from build123d import *

# Parameters (mm, degrees)
BOSS_EXTRUDE1_DEPTH = 20
SHELL1_T            = -5


with BuildPart() as part:
    # Sketch2 → Boss-Extrude1 (new body)
    with BuildSketch(Plane.XY):
        Polygon((-61.336329504, -46.981018343), (97.131391098, -46.981018343), (97.131391098, 27.778459258), (71.904316974, 27.778459258), (71.904316974, 47.185045125), (46.299911218, 47.185045125), (46.299911218, 27.739957348), (-61.336329504, 27.739957348), align=None)
    extrude(amount=BOSS_EXTRUDE1_DEPTH)

    # Shell1
    shell1_openings = [part.faces().sort_by_distance(p)[0] for p in [
        (19.565287633, -7.717892988, 0),
    ]]
    offset(amount=SHELL1_T, openings=shell1_openings, kind=Kind.INTERSECTION)


solid = part.part
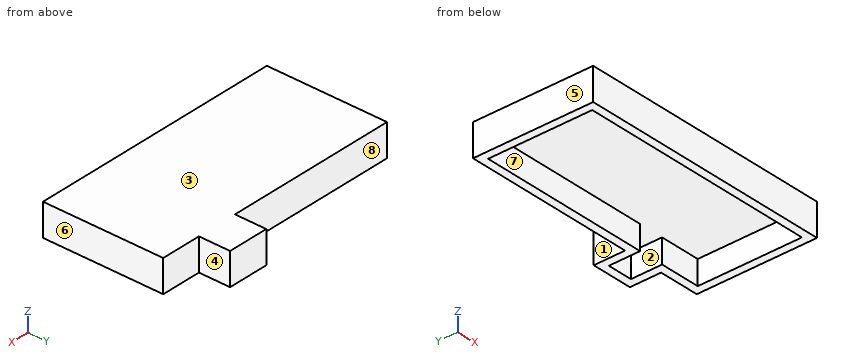
Check sheet for the modelled part. Datum: model origin and axes. Units: mm. Face numbers are marked on the shaded views. A direction names the side the tool comes from. Round coordinates to 2 decimals unless told otherwise and drop trailing zeros. Loops run counter-clockwise (first coordinate to the right, second up) from the corner with the lowest first, then second, coordinate; pieces in that order, holes last. Notation, with made-up numbers: M -32.5,63.25 L 24.5,63.25 A28 cw 24.5,98.25 Z; hole C -10.75,74.25 d6. An arc over 180 degrees is marked long. One line per item, written item: value.
(1) Sectioned sample at B-B, the plane x = 86. Record the cut outline in (y, z).
Computed values:
outline: M -46.98,0 L -41.98,0 L -41.98,15 L 22.78,15 L 22.78,0 L 27.78,0 L 27.78,20 L -46.98,20 Z
(2) Sectioned sample at A-A, the plane y = 34. Record the cut outline in (x, z), then the cut area to 3 significant figures.
Computed values:
outline: M 46.3,0 L 51.3,0 L 51.3,15 L 66.9,15 L 66.9,0 L 71.9,0 L 71.9,20 L 46.3,20 Z
area: 278 mm^2
(3) Depth check by flat-ended pin: pin 1 Ø7.5 at (y, z) = (36, 4.5) entering from -X; pin 2 Ø7.5 at (y, z) = (34, 6) entering from +X; pin 3 Ø12 at (x, z) = (-41.5, 6.5) entering from +Y. Enter the tip coordinate at first touch or a pass-through.
Computed values:
pin 1: stops at x = 46.3
pin 2: stops at x = 71.9
pin 3: stops at y = 27.74
(4) Thickness scan on line 1 (X direction, y = -28.5, z = 6.5); line 2 (Y direction, x = -54, z = 1.5); line 3 (Y direction, x = 89, z = 10.75). Record the ranges inside material, lowest first.
Computed values:
line 1: x = -61.34 to -56.34, 92.13 to 97.13
line 2: y = -46.98 to -41.98, 22.74 to 27.74
line 3: y = -46.98 to -41.98, 22.78 to 27.78
(5) Access from +Z, -Z, +X, -X, +Y, -Y to the whole of each face (thin tool, end or side, straight path). Record for the marked faces 1, 2, 3, 4 and 5.
Computed values:
face 1: +Z, -Z, -X, +Y
face 2: -Z
face 3: +Z, +X, -X, +Y, -Y
face 4: +Z, -Z, +X, +Y
face 5: +Z, -Z, -X, +Y, -Y
(6) Release check for a two-part mould opening along Y. For the marked faces 6, 7 and 8 record: +Y half, -Y half, draft (parallel to the pull), parting line (faces both ways), or undercut.
Computed values:
face 6: draft
face 7: undercut
face 8: +Y half
(7) Sectioned sample at C-C, the plane z = 12.5. Record the cut outline in (x, y).
Computed values:
outline: M -61.34,-46.98 L 97.13,-46.98 L 97.13,27.78 L 71.9,27.78 L 71.9,47.19 L 46.3,47.19 L 46.3,27.74 L -61.34,27.74 Z; hole M -56.34,-41.98 L 92.13,-41.98 L 92.13,22.78 L 66.9,22.78 L 66.9,42.19 L 51.3,42.19 L 51.3,22.74 L -56.34,22.74 Z
